The listing builds one solid part. Answer for the finished solid, in the listing's coordinates (mm). Face numbers are marked on the shaded views. A direction names the side the tool comes from. Coordinates: 2 decimals unless noted, no trailing zeros. Write each loop counter-clockwise with the first axis right and the second up, starting at its lowest first coordinate (ties: lowest second). Pieces come first, ordered by that corner, then holes.
from build123d import *

# Parameters (mm, degrees)
F2_SIZE         = 0.5
F3_R            = 4
F4_DEPTH        = 18.001
F4_COPIES_COUNT = 4


# Not quite as in the source:
# - a pattern or mirror of a feature is missing from the dataset's text; its kind, count and spacing are read off the source's solid


with BuildPart() as f1:
    # F0 (on Front) → F1 (revolve)
    with BuildSketch(Plane.XZ):
        Polygon((-18, 10), (0, 10), (0, 36), (-12, 36), (-12, 20), (-18, 20), align=None)
    revolve(axis=Axis((-9, 0, 0), (1, 0, 0)))

    # F2
    f2_edges = [f1.edges().sort_by_distance(p)[0] for p in [
        (-18, 0, -20),
        (-18, 0, -10),
        (-12, 0, -36),
        (0, 0, -10),
        (0, 0, -36),
    ]]
    chamfer(f2_edges, length=F2_SIZE)

    # F3 (on Right) → F4 (cut, through all)
    with BuildSketch(Plane.YZ):
        with Locations((0, 28)):
            Circle(F3_R)
    f4 = extrude(amount=-F4_DEPTH, mode=Mode.SUBTRACT)

    # F4_copies: F4 ×4 about axis
    f4_copies_axis = Axis((0, 0, 0), (1, 0, 0))
    for i in range(1, F4_COPIES_COUNT):
        add(f4.rotate(f4_copies_axis, i * 360 / F4_COPIES_COUNT), mode=Mode.SUBTRACT)


solid = f1.part
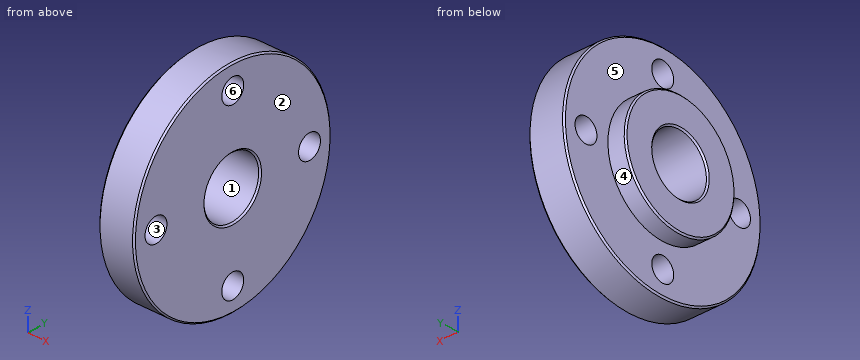
1. For a pull along Y with two mould halves and no side action, classify the marked faces 1, 2, 3 and 4 as pulls with the +Y half, pulls with the -Y half, needs draft (parallel to the pull), parting line crosses it, or undercut.
Results found:
face 1: undercut
face 2: needs draft
face 3: undercut
face 4: parting line crosses it
2. Flat-ended cylindrical pins translate along their axes: P1, Ø6, axis at y = -17, z = 26.5, coming from the +X side; P2, Ø1, axis at y = 22, z = 27, coming from the -X side; P3, Ø4, axis at x = -3.5, z = 6, coming from the -Y side; P4, Ø2, axis at x = -8.5, z = -22, coming from the +Y side. Find the tip coordinate at first contact, or state that the pin passes through.
Results found:
P1: stops at x = 0
P2: stops at x = -12
P3: stops at y = -35.78
P4: stops at y = 29.24
3. Section A-A on z = 0 is taken. State how many separate pieces and enclosed holes the cut face has, then the cut area to 3 significant figures.
Results found:
separate pieces: 4
enclosed holes: 0
area: 551 mm2
4. Section D-D on x = -14.5 is taken. Give the vertices of the cut face in (y, z).
Results found:
outline: circle Ø40 at (0, 0); hole circle Ø20 at (0, 0)
5. Find the intervals of material crossed by L1, parallel to Y at x = -5.5, z = 0; L2, parallel to X at y = 7.5, z = -20, in increasing order.
Results found:
L1: y = -36 to -32, -24 to -10, 10 to 24, 32 to 36
L2: x = -12 to 0
6. A tool of negligible diameter and unlimited length cuts with its end or side. For the marked faces 5 and 6, from which of +Z, -Z, +X, -X, +Y, -Y can it reach the whole face along a straight path? Write none if from no direction.
Results found:
face 5: -X
face 6: +X, -X
7. Section C-C on x = -4.5 is taken. Give the vertices of the cut face in (y, z), then the cut area to 3 significant figures.
Results found:
outline: circle Ø72 at (0, 0); hole circle Ø8 at (-28, 0); hole circle Ø20 at (0, 0); hole circle Ø8 at (0, -28); hole circle Ø8 at (0, 28); hole circle Ø8 at (28, 0)
area: 3,560 mm2
